from build123d import *

# Parameters (mm, degrees)
F0_W     = 30.48
F0_H     = 2.54
F1_DEPTH = 44.45
F0_W_2   = 9.525
F3_DEPTH = 44.45
F4_R     = 2.2225
F5_DEPTH = 25.4
F2_W     = 19.05
F2_H     = 3.175
F6_DEPTH = 25.4
F7_R     = 1.524


# Not quite as in the source:
# - a feature names something its author has since deleted; it is built from what else it names


with BuildPart() as f1:
    # F0 (on Top) → F1 (new body)
    with BuildSketch(Plane.XY):
        with Locations((-15.24, 1.27)):
            Rectangle(F0_W, F0_H)
    extrude(amount=F1_DEPTH)

    # F0 (on Top) → F3 (join)
    with BuildSketch(Plane.XY):
        with Locations((4.7625, 1.27)):
            Rectangle(F0_W_2, F0_H)
    extrude(amount=F3_DEPTH)

    # F4 (on face) + F2 (on face) → F5 (cut)
    with BuildSketch(Plane.XZ):
        with Locations((2.6416, 38.7731)):
            Circle(F4_R)
        with Locations((2.6416, 5.6769)):
            Circle(F4_R)
        with BuildLine():
            Line((9.525, 7.588973174), (9.525, 36.861026826))
            ThreePointArc((9.525, 36.861026826), (1.5875, 22.225), (9.525, 7.588973174))
        make_face()
    with BuildSketch(Plane.XZ):
        with BuildLine():
            Line((-22.098, 9.5885), (-22.098, 12.7635))
            ThreePointArc((-22.098, 12.7635), (-23.8252, 14.4907), (-25.5524, 12.7635))
            Line((-25.5524, 12.7635), (-25.5524, 9.5885))
            ThreePointArc((-25.5524, 9.5885), (-23.8252, 7.8613), (-22.098, 9.5885))
        make_face()
        with BuildLine():
            Line((-22.098, 31.6865), (-22.098, 34.8615))
            ThreePointArc((-22.098, 34.8615), (-23.8252, 36.5887), (-25.5524, 34.8615))
            Line((-25.5524, 34.8615), (-25.5524, 31.6865))
            ThreePointArc((-25.5524, 31.6865), (-23.8252, 29.9593), (-22.098, 31.6865))
        make_face()
        with BuildLine():
            Line((-30.48, 29.337), (-30.48, 15.113))
            ThreePointArc((-30.48, 15.113), (-26.3652, 22.225), (-30.48, 29.337))
        make_face()
    extrude(amount=-F5_DEPTH, mode=Mode.SUBTRACT)

    # F2 (on face) → F6 (cut)
    with BuildSketch(Plane.XZ):
        with Locations((-20.955, 42.8625)):
            Rectangle(F2_W, F2_H)
        with Locations((-20.955, 1.5875)):
            Rectangle(F2_W, F2_H)
    extrude(amount=-F6_DEPTH, mode=Mode.SUBTRACT)

    # F7
    f7_edges = [f1.edges().sort_by_distance(p)[0] for p in [
        (-11.43, 1.27, 41.275),
        (-11.43, 1.27, 44.45),
        (-11.43, 1.27, 0),
        (-11.43, 1.27, 3.175),
    ]]
    fillet(f7_edges, radius=F7_R)


solid = f1.part
Could you check a few things on this model? Use its own coordinates, in mm. A direction names the side the tool comes from. Give positions to 0.01 mm unless a question says otherwise; leave off trailing zeros. Write each loop counter-clockwise with the first axis right and the second up, starting at its lowest first coordinate (ties: lowest second). Pieces come first, ordered by that corner, then holes. Notation, with made-up numbers: (-31.75, 26) -> (16.25, 26) arc R25 ccw to (16.25, 40) -> close; hole circle Ø6 at (51.25, 43.25). An arc over 180 degrees is marked (long way). Answer as CSV lines item,"result". Start each with the question number.
(1) If we section it at A-A, the plane z = 5: Write out the boundary of the cut face in (x, y) (3 decimals), and give its area (3 significant figures).
(2) If we mould it in two halves opening along Z, with no side actions, what happens to faces 5 (the face through (-10.972, 1.288, 44.015)), 6 (the face through (-30.48, 1, 9)), 7 (the face through (-25.552, 1, 33)), 8 (the face through (-23.79, 1.25, 14.49))? For each: +Z half, -Z half, draft (parallel to the pull), parting line (faces both ways), or undercut.
(3) Which directions (+Z, -Z, +X, -X, +Y, -Y) give clear straight access to the entire face, cutting with the end or side of a thin tool? Please do faces 1 (the face through (0, 1, 44.45)), 2 (the face through (-22, 1, 41.275)), 3 (the face through (-22.098, 1, 11)), 4 (the face through (-22, 1, 3.175)).
(4) If we section it at D-D, the plane z = 21: Write out the boundary of the cut face in (x, y), and give its area (3 significant figures).
(5) I'm going to push flat-ended pins straight in: pin 1 Ø0.8 at (x, y) = (-22, 1.5) entering from +Z (3 decimals); pin 2 Ø2.5 at (x, z) = (2.64, 38.77) entering from +Y; pin 3 Ø0.8 at (x, y) = (-23, 1.5) entering from -Z (3 decimals); pin 4 Ø1.5 at (x, z) = (-13, 19) entering from -Y. Where does each tip first touch, or does it pass through?
(6) Please list where these lines run through material, in increasing order: line 1 (Z direction, x = -23, y = 0.7) (3 decimals); line 2 (Z direction, x = 4, y = 0.9); line 3 (Z direction, x = -24.5, y = 1.2) (3 decimals).
(7) If we section it at C-C, the plane x = 1: Write out the boundary of the cut face in (y, z).
(8) If we section it at B-B, the plane y = 1.95: Give the number of separate pieces and of enclosed holes in the cut face, and give its area (3 significant figures).
Answer list:
1,outline,"(-30.48, 0) -> (0.525, 0) -> (0.525, 2.54) -> (-30.48, 2.54) -> close; (4.759, 0) -> (9.525, 0) -> (9.525, 2.54) -> (4.759, 2.54) -> close"
1,area,"90.9 mm^2"
2,face 5,"+Z half"
2,face 6,"draft"
2,face 7,"undercut"
2,face 8,"undercut"
3,face 1,"+Z, +X, -X, +Y, -Y"
3,face 2,"+Z, -X, +Y, -Y"
3,face 3,"+Y, -Y"
3,face 4,"-Z, -X, +Y, -Y"
4,outline,"(-26.46, 0) -> (1.63, 0) -> (1.63, 2.54) -> (-26.46, 2.54) -> close"
4,area,"71.3 mm^2"
5,pin 1,"z = 41.275"
5,pin 2,"through"
5,pin 3,"z = 3.175"
5,pin 4,"y = 0"
6,line 1,"3.175 to 8.071, 14.281 to 30.169, 36.379 to 41.275"
6,line 2,"0 to 3.92, 7.44 to 13.37, 31.08 to 37.01, 40.53 to 44.45"
6,line 3,"3.175 to 7.999, 14.353 to 30.097, 36.451 to 41.275"
7,outline,"(0, 0) -> (2.54, 0) -> (2.54, 4.18) -> (0, 4.18) -> close; (0, 7.18) -> (2.54, 7.18) -> (2.54, 37.27) -> (0, 37.27) -> close; (0, 40.27) -> (2.54, 40.27) -> (2.54, 44.45) -> (0, 44.45) -> close"
8,separate pieces,"1"
8,enclosed holes,"4"
8,area,"1,380 mm^2"
